```python
from build123d import *

# Parameters (mm, degrees)
F0_W     = 4.3434
F0_H     = 101.6
F1_DEPTH = 25.4
F2_W     = 4.3434
F2_H     = 4.3434
F3_DEPTH = 25.401


with BuildPart() as f1:
    # F0 (on Top) → F1 (new body)
    with BuildSketch(Plane.XY):
        Polygon((67.536269, 49.751887), (-41.683737, 49.751887), (-41.683737, -13.240114), (7.084264, -13.240114), (11.427664, -13.240114), (67.536269, -13.240114), align=None)
        with Locations((9.255964, -64.040114)):
            Rectangle(F0_W, F0_H)
    extrude(amount=F1_DEPTH)

    # F2 (on face) → F3 (cut, through all)
    with BuildSketch(Plane.XY.offset(25.4)):
        with Locations((12.330785, 4.937064)):
            Rectangle(F2_W, F2_H)
    extrude(amount=-F3_DEPTH, mode=Mode.SUBTRACT)


solid = f1.part
```
Input: part model. Units: mm. Frame: model coordinates. A direction names the side the tool comes from. Give positions to 0.01 mm unless a question says otherwise; leave off trailing zeros. Order: outer loops, then holes, each group sorted by start corner. A loop starts at its lowest first (then second) coordinate and runs counter-clockwise, first axis right, second up.
1. Section B-B on x = 2.5. Return the cut outline in (y, z).
Derived:
outline: (-13.24, 0) - (49.75, 0) - (49.75, 25.4) - (-13.24, 25.4) - close
2. Pin query (flat end, axial travel): pin 1 (7.5 mm diameter, centred on y = -60, z = 11.5, fed in from -X); pin 2 (1 mm diameter, centred on x = 42.5, z = 10, fed in from -Y). Return the tip coordinate at first contact, or that it passes through.
Derived:
pin 1: stops at x = 7.08
pin 2: stops at y = -13.24
3. Section A-A on z = 9.5. Return the cut outline in (x, y).
Derived:
outline: (-41.68, -13.24) - (7.08, -13.24) - (7.08, -114.84) - (11.43, -114.84) - (11.43, -13.24) - (67.54, -13.24) - (67.54, 49.75) - (-41.68, 49.75) - close; hole (10.16, 2.77) - (14.5, 2.77) - (14.5, 7.11) - (10.16, 7.11) - close
4. Reachability of faces 4 (the flat face through (12, 23, 25.4)), 5 (the flat face through (7.084, -65, 13)), 6 (the flat face through (12, 7.109, 13)) from +Z, -Z, +X, -X, +Y, -Y: full face, straight path, thin tool, end or side. Return the list, or none.
Derived:
face 4: +Z, +X, -X, +Y, -Y
face 5: +Z, -Z, -X, -Y
face 6: +Z, -Z
5. Material intervals for L1, parallel to X at y = -21, z = 21.25; L2, parallel to Y at x = -30.5, z = 12.75; L3, parallel to Y at x = 10.5, z = 20.5, sorted ascending.
Derived:
L1: x = 7.08 to 11.43
L2: y = -13.24 to 49.75
L3: y = -114.84 to 2.77, 7.11 to 49.75
6. Section C-C on y = -40. Return the cut outline in (x, z).
Derived:
outline: (7.08, 0) - (11.43, 0) - (11.43, 25.4) - (7.08, 25.4) - close
7. Mould query, pull axis Y, two halves, no side actions, for faces 1 (the flat face through (11.428, -65, 13)), 2 (the flat face through (39, -13.24, 13)), 3 (the flat face through (10.159, 5, 13)). Classes: released by +Y, released by -Y, zero draft, split by the parting line, or undercut.
Derived:
face 1: zero draft
face 2: released by -Y
face 3: undercut
